```python
from build123d import *

# Parameters (mm, degrees)
SKETCH1_W           = 203.2
SKETCH1_H           = 203.2
BOSS_EXTRUDE1_DEPTH = 38.1
SKETCH2_R           = 25.4
CUT_EXTRUDE1_DEPTH  = 12.7
SKETCH3_R           = 19.05
CUT_EXTRUDE2_DEPTH  = 146.911891222


with BuildPart() as part:
    # Sketch1 → Boss-Extrude1 (new body)
    with BuildSketch(Plane.XZ):
        Rectangle(SKETCH1_W, SKETCH1_H)
    extrude(amount=BOSS_EXTRUDE1_DEPTH)

    # Sketch2 → Cut-Extrude1 (cut)
    with BuildSketch(Plane(origin=(0, 0, 0), x_dir=(1, 0, 0), z_dir=(0, 1, 0))):
        with Locations(Location((0, 0, 0), (0, 0, 270))):
            Circle(SKETCH2_R)
    extrude(amount=-CUT_EXTRUDE1_DEPTH, mode=Mode.SUBTRACT)

    # Sketch3 → Cut-Extrude2 (cut, through all)
    with BuildSketch(Plane(origin=(0, -12.7, 0), x_dir=(1, 0, 0), z_dir=(0, 1, 0))):
        with Locations(Location((0, 0, 0), (0, 0, 270))):
            Circle(SKETCH3_R)
    extrude(amount=-CUT_EXTRUDE2_DEPTH, mode=Mode.SUBTRACT)


solid = part.part
```
Input: part model. Units: mm. Frame: model coordinates. A direction names the side the tool comes from. Round coordinates to 2 decimals unless told otherwise and drop trailing zeros. Loops run counter-clockwise (first coordinate to the right, second up) from the corner with the lowest first, then second, coordinate; pieces in that order, holes last. Notation, with made-up numbers: (74, 51) -> (113, 51) arc R29 cw to (113, 81) -> close; hole circle Ø4 at (61, -35.5). An arc over 180 degrees is marked (long way). One line per item, written item: value.
(1) Section B-B (x = 0). Return the cut outline in (y, z), plus the area to 3 significant figures.
Geometry check:
outline: (-38.1, -101.6) -> (0, -101.6) -> (0, -25.4) -> (-12.7, -25.4) -> (-12.7, -19.05) -> (-38.1, -19.05) -> close; (-38.1, 19.05) -> (-12.7, 19.05) -> (-12.7, 25.4) -> (0, 25.4) -> (0, 101.6) -> (-38.1, 101.6) -> close
area: 6,130 mm2
(2) Mould query, pull axis Z, two halves, no side actions, for faces 1 (the face through (101.6, -19, -1)), 2 (the face through (-1, -19, -101.6)), 3 (the face through (-11.59, -25.22, -15.12)), 4 (the face through (19, -12.7, 4)). Classes: pulls with the +Z half, pulls with the -Z half, needs draft (parallel to the pull), parting line crosses it, or undercut.
Geometry check:
face 1: needs draft
face 2: pulls with the -Z half
face 3: undercut
face 4: undercut
(3) Material intervals for line 1 (X direction, y = -8, z = 0); line 2 (X direction, y = -20, z = 0); line 3 (Z direction, x = -15.5, y = -35), sorted ascending. Write a range as [from, to].
Geometry check:
line 1: [-101.6, -25.4], [25.4, 101.6]
line 2: [-101.6, -19.05], [19.05, 101.6]
line 3: [-101.6, -11.07], [11.07, 101.6]
(4) Section C-C (y = -8.5). Return the cut outline in (x, z), plus the area to 3 significant figures.
Geometry check:
outline: (-101.6, -101.6) -> (101.6, -101.6) -> (101.6, 101.6) -> (-101.6, 101.6) -> close; hole circle Ø50.8 at (0, 0)
area: 39,300 mm2
(5) Section A-A (z = 0). Return the cut outline in (x, y).
Geometry check:
outline: (-101.6, -38.1) -> (-19.05, -38.1) -> (-19.05, -12.7) -> (-25.4, -12.7) -> (-25.4, 0) -> (-101.6, 0) -> close; (19.05, -38.1) -> (101.6, -38.1) -> (101.6, 0) -> (25.4, 0) -> (25.4, -12.7) -> (19.05, -12.7) -> close
(6) Set-up query: faces 5 (the face through (-1, -19, 101.6)), 6 (the face through (-15.456, -6.261, -20.157)). Return all of +Z, -Z, +X, -X, +Y, -Y with unobstructed straight access to the full face (end or side cutting, diameter ignored); none if empty.
Geometry check:
face 5: +Z, +X, -X, +Y, -Y
face 6: +Y
